CAD build for the part. Positions are in the model's coordinates, mm. Face numbers are marked on the shaded views. A direction names the side the tool comes from. Give positions to 0.01 mm unless a question says otherwise; leave off trailing zeros. Write each loop counter-clockwise with the first axis right and the second up, starting at its lowest first coordinate (ties: lowest second). Pieces come first, ordered by that corner, then holes. Notation, with made-up numbers: M -4.75,-22.75 L 12.25,-22.75 A34 cw 12.25,7.25 Z; hole C -16.5,-35 d5. An arc over 180 degrees is marked long. One line per question, with ' | ' between items. Start each with the question number.
1. Cut at D-D, the plane z = 0. Count the separate pieces of the cut face and the enclosed holes in it, then the cut area to 3 significant figures.
2. Cut at B-B, the plane y = 2.25. Write the cut outline in (x, z) (1 decimal).
3. Cut at A-A, the plane x = 1.5. Write the cut outline in (y, z) (3 decimals).
4. Pull direction Y, two halves, no side cores. Call the marked faces 6, 7 and 8: released by +Y, released by -Y, zero draft, split by the parting line, or undercut.
5. Wall check: L1, parallel to X at y = -1, z = 1; L2, parallel to Y at x = 7.45, z = 0; L3, parallel to X at y = 2.75, z = 2.5. Give the ranges that are in metal, low to high.
6. Flat gauge pins, fed straight in: pin 1 (2 mm diameter, centred on x = -4.5, z = 1.5, fed in from -Y); pin 2 (0.6 mm diameter, centred on x = 7.5, y = -1.5, fed in from +Z); pin 3 (1 mm diameter, centred on y = 11, z = 0.5, fed in from +X). Where does each tip first touch, or does it go through?
7. Cut at C-C, the plane z = 2.5. Write the cut outline in (x, y).
8. Which spindle directions (+Z, -Z, +X, -X, +Y, -Y) get a long thin tool onto all of the face, cutting with end or side? Do the marked faces 1, 2, 3, 4 and 5. Say none if no direction does.
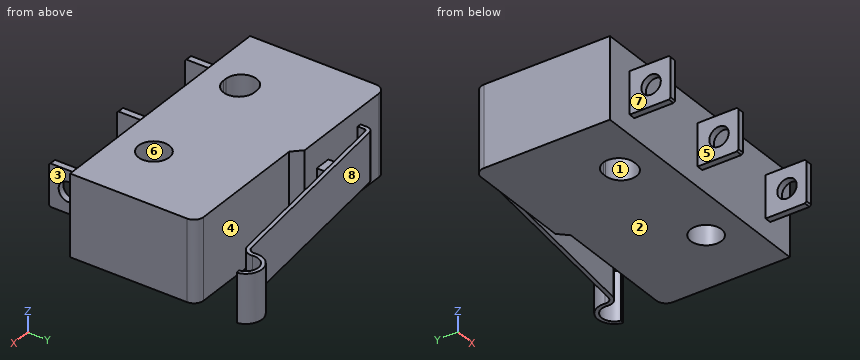
```python
from build123d import *

# Parameters (mm, degrees)
SKETCH2_R           = 1.2065
EXTRUDE1_DEPTH      = 3.175
EXTRUDE2_DEPTH      = 1.1049
SKETCH10_R          = 0.762
EXTRUDE6_DEPTH      = 0.254
LPATTERN1_COUNT     = 3
LPATTERN1_PITCH     = 7.493
EXTRUDE_THIN1_DEPTH = 1.905


with BuildPart() as part:
    # Sketch2 → Extrude1 (new body, symmetric)
    with BuildSketch(Plane.XY):
        with BuildLine():
            Line((-9.1567, 10.6172), (-4.9149, 10.6172))
            Line((-4.9149, 10.6172), (-0.9779, 10.6172))
            Line((-0.9779, 10.6172), (-0.2667, 9.906))
            Line((-0.2667, 9.906), (9.1567, 9.906))
            ThreePointArc((9.1567, 9.906), (9.695515367, 9.682815367), (9.9187, 9.144))
            Line((9.9187, 9.144), (9.9187, 0))
            Line((9.9187, 0), (-9.9187, 0))
            Line((-9.9187, 0), (-9.9187, 9.8552))
            ThreePointArc((-9.9187, 9.8552), (-9.695515367, 10.394015367), (-9.1567, 10.6172))
        make_face()
        with Locations((4.7117, 2.8575)):
            Circle(SKETCH2_R, mode=Mode.SUBTRACT)
        with BuildLine():
            Line((-4.9149, 4.064), (-4.6609, 4.064))
            ThreePointArc((-4.6609, 4.064), (-3.4544, 2.8575), (-4.6609, 1.651))
            Line((-4.6609, 1.651), (-4.9149, 1.651))
            ThreePointArc((-4.9149, 1.651), (-6.1214, 2.8575), (-4.9149, 4.064))
        make_face(mode=Mode.SUBTRACT)
    extrude(amount=EXTRUDE1_DEPTH, both=True)

    # Sketch10 → Extrude6 (add, symmetric)
    with BuildSketch(Plane(origin=(-7.493, 0, 0), x_dir=(0, 0, -1), z_dir=(1, 0, 0))):
        Polygon((-1.651, 0), (-1.651, -3.0734), (-1.524, -3.2004), (1.524, -3.2004), (1.651, -3.0734), (1.651, 0), align=None)
        with Locations((0, -1.6764)):
            Circle(SKETCH10_R, mode=Mode.SUBTRACT)
    extrude6 = extrude(amount=EXTRUDE6_DEPTH, both=True)

    # LPattern1: Extrude6 ×3
    with Locations(*[(i * LPATTERN1_PITCH, 0, 0) for i in range(1, LPATTERN1_COUNT)]):
        add(extrude6)



with BuildPart() as body_2:
    # Sketch3 → Extrude2 (new body, symmetric)
    with BuildSketch(Plane.XY):
        with BuildLine():
            Line((-3.5814, 10.6172), (-3.5814, 11.524614746))
            ThreePointArc((-3.5814, 11.524614746), (-2.9464, 11.7475), (-2.3114, 11.524614746))
            Line((-2.3114, 11.524614746), (-2.3114, 10.6172))
            Line((-2.3114, 10.6172), (-3.5814, 10.6172))
        make_face()
    extrude(amount=EXTRUDE2_DEPTH, both=True)


with BuildPart() as part_1:
    add(part.part)

    add(body_2.part)  # Extrude-Thin1 merges body 2
    # Sketch11 → Extrude-Thin1 (add, symmetric)
    with BuildSketch(Plane.XY):
        with BuildLine():
            Line((-7.1247, 10.6172), (-7.1247, 11.128280087))
            ThreePointArc((-7.1247, 11.128280087), (-6.995143389, 11.467167386), (-6.672555901, 11.6332))
            Line((-6.672555901, 11.6332), (8.711185108, 13.335))
            ThreePointArc((8.711185108, 13.335), (9.057341476, 13.529355692), (9.157991006, 13.913371366))
            ThreePointArc((9.157991006, 13.913371366), (10.231016869, 15.353654497), (11.6713, 14.280628634))
            Line((11.6713, 14.280628634), (11.369702921, 14.236557762))
            ThreePointArc((11.369702921, 14.236557762), (10.275087741, 15.052057418), (9.459588085, 13.957442238))
            ThreePointArc((9.459588085, 13.957442238), (9.298548838, 13.343017159), (8.744698648, 13.032048052))
            Line((8.744698648, 13.032048052), (-6.63904236, 11.330248052))
            ThreePointArc((-6.63904236, 11.330248052), (-6.768077356, 11.263835007), (-6.8199, 11.128280087))
            Line((-6.8199, 11.128280087), (-6.8199, 10.6172))
            Line((-6.8199, 10.6172), (-7.1247, 10.6172))
        make_face()
    extrude(amount=EXTRUDE_THIN1_DEPTH, both=True)


solid = part_1.part
```
Here are the results:
1) separate pieces: 4 | enclosed holes: 3 | area: 203 mm^2
2) outline: M -9.9,-3.2 L -6,-3.2 L -6,3.2 L -9.9,3.2 Z; M -3.6,-3.2 L 3.7,-3.2 L 3.7,3.2 L -3.6,3.2 Z; M 5.8,-3.2 L 9.9,-3.2 L 9.9,3.2 L 5.8,3.2 Z
3) outline: M 0,-3.175 L 9.906,-3.175 L 9.906,3.175 L 0,3.175 Z; M 12.231,-1.905 L 12.537,-1.905 L 12.537,1.905 L 12.231,1.905 Z
4) face 6: undercut | face 7: zero draft | face 8: released by +Y
5) L1: -7.75 to -7.24, -0.25 to 0.25, 7.24 to 7.75 | L2: -3.2 to -2.44, -0.91 to 9.91, 12.89 to 13.2 | L3: -9.92 to -6.12, -3.46 to 3.51, 5.91 to 9.92
6) pin 1: y = 0 | pin 2: z = 1.65 | pin 3: x = -0.86
7) outline: M -9.92,0 L 9.92,0 L 9.92,9.14 A0.76 ccw 9.16,9.91 L -0.27,9.91 L -0.98,10.62 L -9.16,10.62 A0.76 ccw -9.92,9.86 Z; hole M -4.91,1.65 L -4.66,1.65 A1.21 ccw -4.66,4.06 L -4.91,4.06 A1.21 ccw Z; hole C 4.71,2.86 d2.41
8) face 1: +Z, -Z | face 2: -Z, +X, -X, +Y, -Y | face 3: +Z, -Z, +X, -Y | face 4: +Z, -Z, +X | face 5: +Z, -Z, -Y
